```python
from build123d import *

# Parameters (mm, degrees)
SKETCH_22_R              = 43
EXTRUDE_5_DEPTH          = 17
SKETCH_24_R              = 22.244
EXTRUDE_6_DEPTH          = 5
SKETCH_25_R              = 32.76
CUT_EXTRUDE_9_DEPTH      = 15
SKETCH_26_R              = 12.5
CUT_EXTRUDE_10_DEPTH     = 10
SKETCH_27_R              = 2.7
CUT_EXTRUDE_11_DEPTH     = 6.1
PATTERN_CIRCULAR_6_COUNT = 6
SKETCH_29_R              = 2.2
CUT_EXTRUDE_12_DEPTH     = 64.14269554
PATTERN_CIRCULAR_7_COUNT = 6


with BuildPart() as part:
    # 스케치22 → 보스-돌출5 (new body)
    with BuildSketch(Plane(origin=(0, 0, 0), x_dir=(1, 0, 0), z_dir=(0, 1, 0))):
        with Locations(Location((0, 0, 0), (0, 0, 270))):
            Circle(SKETCH_22_R)
    extrude(amount=EXTRUDE_5_DEPTH)

    # 스케치24 → 보스-돌출6 (add)
    with BuildSketch(Plane(origin=(0, 17, 0), x_dir=(1, 0, 0), z_dir=(0, 1, 0))):
        with Locations(Location((0, 0, 0), (0, 0, 270))):
            Circle(SKETCH_24_R)
    extrude(amount=EXTRUDE_6_DEPTH)

    # 스케치25 → 컷-돌출9 (cut)
    with BuildSketch(Plane.XZ):
        with Locations(Location((0, 0, 0), (0, 0, 270))):
            Circle(SKETCH_25_R)
    extrude(amount=-CUT_EXTRUDE_9_DEPTH, mode=Mode.SUBTRACT)

    # 스케치26 → 컷-돌출10 (cut)
    with BuildSketch(Plane(origin=(0, 22, 0), x_dir=(1, 0, 0), z_dir=(0, 1, 0))):
        with Locations(Location((0, 0, 0), (0, 0, 270))):
            Circle(SKETCH_26_R)
    extrude(amount=-CUT_EXTRUDE_10_DEPTH, mode=Mode.SUBTRACT)

    # 스케치27 → 컷-돌출11 (cut)
    with BuildSketch(Plane(origin=(0, 22, 0), x_dir=(1, 0, 0), z_dir=(0, 1, 0))):
        with Locations(Location((0, 17.5, 0), (0, 0, 270))):
            Circle(SKETCH_27_R)
    cut_extrude_11 = extrude(amount=-CUT_EXTRUDE_11_DEPTH, mode=Mode.SUBTRACT)

    # 원형 패턴6: 컷-돌출11 ×6 about axis
    pattern_circular_6_axis = Axis((0, 0, 0), (0, 1, 0))
    for i in range(1, PATTERN_CIRCULAR_6_COUNT):
        add(cut_extrude_11.rotate(pattern_circular_6_axis, i * 360 / PATTERN_CIRCULAR_6_COUNT), mode=Mode.SUBTRACT)

    # 스케치29 → 컷-돌출12 (cut, through all)
    with BuildSketch(Plane(origin=(0, 17, 0), x_dir=(1, 0, 0), z_dir=(0, 1, 0))):
        with Locations(Location((0, 37, 0), (0, 0, 270))):
            Circle(SKETCH_29_R)
    cut_extrude_12 = extrude(amount=-CUT_EXTRUDE_12_DEPTH, mode=Mode.SUBTRACT)

    # 원형 패턴7: 컷-돌출12 ×6 about axis
    pattern_circular_7_axis = Axis((0, 0, 0), (0, 1, 0))
    for i in range(1, PATTERN_CIRCULAR_7_COUNT):
        add(cut_extrude_12.rotate(pattern_circular_7_axis, i * 360 / PATTERN_CIRCULAR_7_COUNT), mode=Mode.SUBTRACT)


solid = part.part
```
Geometry: final body of the model. Coordinates: model frame, mm. A direction names the side the tool comes from. Give positions to 0.01 mm unless a question says otherwise; leave off trailing zeros. Order: outer loops, then holes, each group sorted by start corner. A loop starts at its lowest first (then second) coordinate and runs counter-clockwise, first axis right, second up. Notation, with made-up numbers: (-17.75, 64) -> (34.25, 64) arc R28 ccw to (34.25, 97) -> close; hole circle Ø9 at (24.25, 83.5). An arc over 180 degrees is marked (long way). Write each question's results on one line, items separated by ' | '. Start each with the question number.
1) First-contact query: pin 1 (6 mm diameter, centred on x = -15.16, z = -8.75, fed in from -Y); pin 2 (1.5 mm diameter, centred on x = -20, y = 4, fed in from -Z); pin 3 (6 mm diameter, centred on x = -8.5, y = 17, fed in from +Z). Flat tips, straight axial feed; report the tip coordinate or a pass-through.
2) Section A-A (z = 0). Return loops of the section in (x, y), then the cut area to 3 significant figures.
3) Section C-C (y = 8.5). Return loops of the section in (x, z).
4) Set-up query: faces 1 (the cylindrical face through (-0.097, 8.619, 39.198)), 2 (the cylindrical face through (13.33, 18.99, -6.76)), 3 (the cylindrical face through (-19.93, 7.4, 26)). Return all of +Z, -Z, +X, -X, +Y, -Y with unobstructed straight access to the full face (end or side cutting, diameter ignored); none if empty.
5) Draft query along Z for faces 4 (the cylindrical face through (0.097, 8.619, -39.198)), 5 (the flat face through (-10, 22, 10)), 6 (the cylindrical face through (18.756, 19.465, 11.958)). Return one class per face: pulls with the +Z half, pulls with the -Z half, needs draft (parallel to the pull), parting line crosses it, or undercut.
6) Section D-D (x = -28.5). Return loops of the section in (y, z), then the cut area to 3 significant figures.
7) Line query: line 1 (Z direction, x = 33.5, y = 4.75); line 2 (Z direction, x = 14, y = 19); line 3 (X direction, y = 15.25, z = -19). Output: solid intervals per line, ascending. Write a range as from..to.
8) Section B-B (x = -4.5). Return loops of the section in (y, z).
Calculated:
1) pin 1: y = 15 | pin 2: z = -38.45 | pin 3: z = 42.65
2) outline: (-43, 0) -> (-32.76, 0) -> (-32.76, 15) -> (-12.5, 15) -> (-12.5, 22) -> (-22.24, 22) -> (-22.24, 17) -> (-43, 17) -> close; (12.5, 15) -> (32.76, 15) -> (32.76, 0) -> (43, 0) -> (43, 17) -> (22.24, 17) -> (22.24, 22) -> (12.5, 22) -> close | area: 527 mm2
3) outline: circle Ø86 at (0, 0); hole circle Ø4.4 at (-32.04, -18.5); hole circle Ø4.4 at (-32.04, 18.5); hole circle Ø65.52 at (0, 0); hole circle Ø4.4 at (0, -37); hole circle Ø4.4 at (0, 37); hole circle Ø4.4 at (32.04, -18.5); hole circle Ø4.4 at (32.04, 18.5)
4) face 1: +Y, -Y | face 2: +Y | face 3: -Y
5) face 4: undercut | face 5: needs draft | face 6: parting line crosses it
6) outline: (0, -32.2) -> (17, -32.2) -> (17, 32.2) -> (0, 32.2) -> (0, 16.15) -> (15, 16.15) -> (15, -16.15) -> (0, -16.15) -> close | area: 610 mm2
7) line 1: -26.96..-20.15, -16.85..16.85, 20.15..26.96 | line 2: -17.29..-11.19, -6.31..6.31, 11.19..17.29 | line 3: -38.57..-34.19, -29.9..29.9, 34.19..38.57
8) outline: (0, -42.76) -> (17, -42.76) -> (17, -21.78) -> (22, -21.78) -> (22, -11.66) -> (15, -11.66) -> (15, -32.45) -> (0, -32.45) -> close; (0, 32.45) -> (15, 32.45) -> (15, 11.66) -> (22, 11.66) -> (22, 21.78) -> (17, 21.78) -> (17, 42.76) -> (0, 42.76) -> close
